Print and shaded views of the part. All mm, measured from the part's lowest x, y and z. Round coordinates to 2 decimals unless told otherwise and drop trailing zeros. Write each loop counter-clockwise with the first axis right and the second up, starting at its lowest first coordinate (ties: lowest second). Pieces come first, ordered by that corner, then holes. Notation, with made-up numbers: M 38.5,-39 L 80.5,-39 A16 cw 80.5,-15 Z; hole C 88.25,22.5 d6. An arc over 180 degrees is marked long. Write item = value, one per line. Start each with the question number.
Q1. Probe L1, parallel to Y at x = 2.65, z = 54.5 (1 decimal); L2, parallel to Z at x = 0.55, y = 2.5 (1 decimal). List the from-to ranges inside material, lowest first.
Q2. Band-saw the part on B-B on z = 51.5. Write the cut outline in (x, y) (1 decimal), plus the area to 3 significant figures.
Q3. Drop a flat-ended pin along its axis: P1, Ø1, axis at x = 2.5, z = 3, coming from the -Y side (3 decimals). Give the stop position or say it passes through.
Q4. Band-saw the part on A-A on x = 2.6. Write the cut outline in (y, z) (1 decimal), plus the area to 3 significant figures.
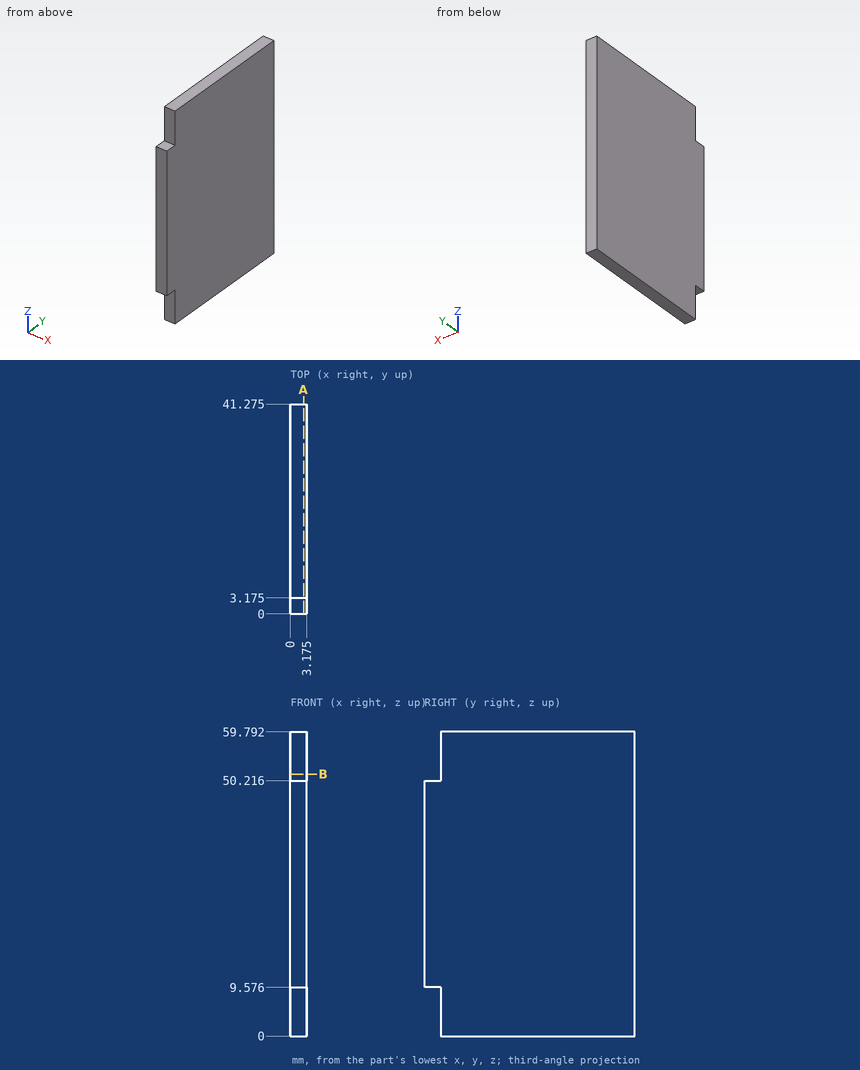
Conclusion:
q1.L1 = 3.2 to 41.3
q1.L2 = 9.6 to 50.2
q2.outline = M 0,3.2 L 3.2,3.2 L 3.2,41.3 L 0,41.3 Z
q2.area = 121 mm^2
q3.P1 = 3.175
q4.outline = M 0,9.6 L 3.2,9.6 L 3.2,0 L 41.3,0 L 41.3,59.8 L 3.2,59.8 L 3.2,50.2 L 0,50.2 Z
q4.area = 2,410 mm^2
